Answer from the drawing. Dimensions are ordinates in mm from the lowest x, y and z of the part. Give positions to 0.01 mm unless a question says otherwise; leave off trailing zeros. Loops run counter-clockwise (first coordinate to the right, second up) from the corner with the lowest first, then second, coordinate; pieces in that order, holes last. Notation, with made-up numbers: (0, -29.75) - (28, -29.75) arc R31 ccw to (28, 7.25) - close; hole circle Ø5 at (86.5, 49.5). An arc over 180 degrees is marked (long way). Put each result on its own line as item: value. Start each with the question number.
1. A cutting plane is placed at C-C, the plane x = 122. Determine the outline of the cut face in (y, z) (1 decimal), plus the area to 3 significant figures.
2. Consider L1, parallel to X at y = 79, z = 1.25; L2, parallel to X at y = 96, z = 2.4; L3, parallel to Y at x = 123, z = 2.6 (1 decimal). Determine where each line is inside the solid, lowest interval first. Write a range as from..to.
3. A cutting plane is placed at B-B, the plane y = 71.5. Determine the outline of the cut face in (x, z) (1 decimal).
4. Given pin 1 Ø1 at (y, z) = (151.5, 2) entering from -X; pin 2 Ø0.9 at (y, z) = (90.5, 1) entering from +X; pin 3 Ø1.5 at (x, z) = (91.5, 1.5) entering from -Y, each flat-ended and moving along its own axis, determine where each tip first touches the part or whether it passes through.
5. A cutting plane is placed at A-A, the plane z = 1.1. Determine the outline of the cut face in (x, y), plus the area to 3 significant figures.
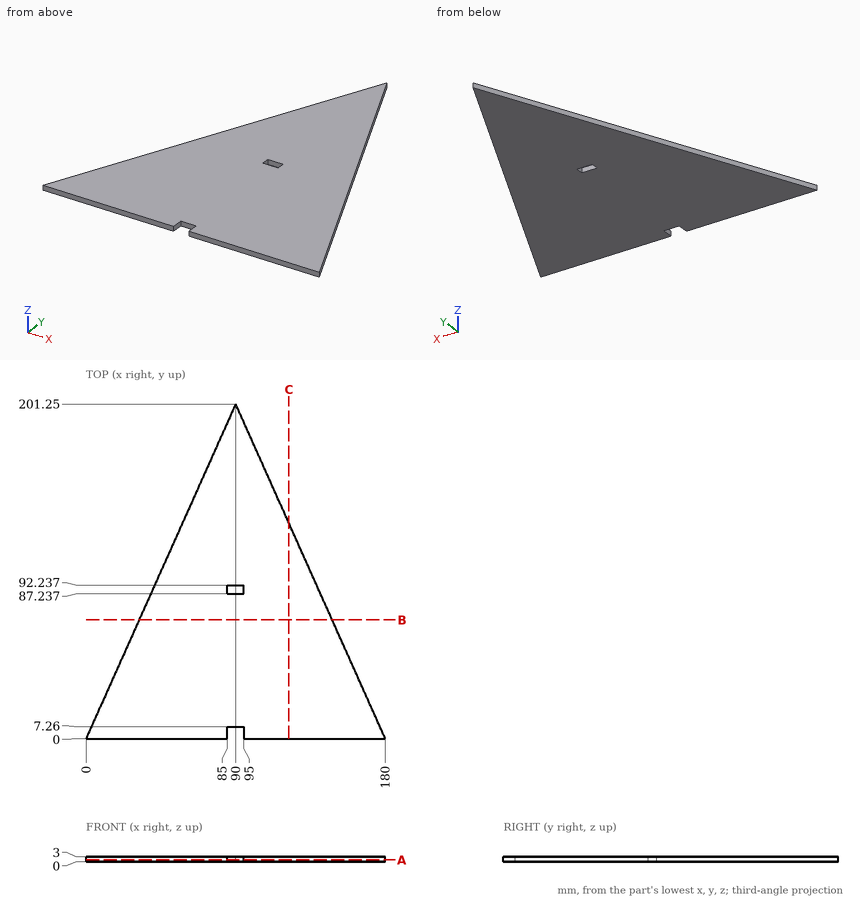
Return value:
1. outline: (0, 0) - (129.7, 0) - (129.7, 3) - (0, 3) - close
1. area: 389 mm2
2. L1: x = 35.33..144.67
2. L2: x = 42.93..137.07
2. L3: y = 0..127.5
3. outline: (32, 0) - (148, 0) - (148, 3) - (32, 3) - close
4. pin 1: stops at x = 67.53
4. pin 2: stops at x = 139.73
4. pin 3: stops at y = 7.26
5. outline: (0, 0) - (85, 0) - (85, 7.26) - (95, 7.26) - (95, 0) - (180, 0) - (90, 201.25) - close; hole (85, 87.24) - (95, 87.24) - (95, 92.24) - (85, 92.24) - close
5. area: 18,000 mm2
